Work out the finished part from the listing and answer in its coordinate system (mm). Coordinates: 2 decimals unless noted, no trailing zeros. Write each loop counter-clockwise with the first axis right and the second up, starting at its lowest first coordinate (ties: lowest second). Pieces come first, ordered by that corner, then holes. Notation, with made-up numbers: (-27, 17.25) - (4, 17.25) arc R5 cw to (4, 26.25) - close; hole circle Ø9 at (50.5, 54.25). An arc over 180 degrees is marked (long way). Use a Markdown table: item, result. Add a question column.
(1) The part is cut by section A-A, the plane z = 38.1. Give the vertices of the cut face in (x, y) (3 decimals).
(2) For a pull along X with two mould halves and no side action, classify faces 1 (the face through (-15.075, -0.044, -1.252)), 2 (the face through (-19, 0, -57.15)), 3 (the face through (38.1, 0, 38)), 4 (the face through (-19.592, -0.044, -42.232)) as released by +X, released by -X, zero draft, split by the parting line, or undercut.
(3) The part is cut by section C-C, the plane y = 0. Give the vertices of the cut face in (x, z).
(4) Find the intervals of material crossed by line 1 (Z direction, x = -19.05, y = 1); line 2 (X direction, y = -0.5, z = 38.1); line 3 (Z direction, x = -21, y = -1.5), in increasing order. Write a range as from..to.
(5) The part is cut by section B-B, the plane x = -19.05. Give the vertices of the cut face in (y, z) (3 decimals).
(6) The part is cut by section D-D, the plane x = 19.05. Give the vertices of the cut face in (y, z) (3 decimals), then the cut area to 3 significant figures.
(7) Given pin 1 Ø3 at (x, y) = (13.5, -1.5) entering from -Z; pin 2 Ø3 at (y, z) = (0, -25) entering from +X (3 decimals), each flat-ended and moving along its own axis, determine where each tip first touches the part or whether it passes through.
from build123d import *

# Parameters (mm, degrees)
SKETCH1_W           = 76.2
SKETCH1_H           = 6.35
BOSS_EXTRUDE1_DEPTH = 57.15
CUT_EXTRUDE3_DEPTH  = 7.62
LPATTERN1_START     = -3.175
LPATTERN1_OUTLINE_R = 4.167251
LPATTERN1_DEPTH     = 6.35


# Read off the part's stored shape, not the designer's step: LPattern1
with BuildPart() as part:
    # Sketch1 → Boss-Extrude1 (new, symmetric)
    with BuildSketch(Plane.XY):
        Rectangle(SKETCH1_W, SKETCH1_H)
    extrude(amount=BOSS_EXTRUDE1_DEPTH, both=True)

    # Sketch8 → Cut-Extrude3 (cut)
    with BuildSketch(Plane(origin=(0, 3.175, 0), x_dir=(-1, 0, 0), z_dir=(0, 1, 0))):
        Polygon((0, -57.15), (-38.1, 19.05), (-38.1, -57.15), align=None)
    extrude(amount=-CUT_EXTRUDE3_DEPTH, mode=Mode.SUBTRACT)

    # Sketch9 → 21_64 _0.32813_ Diameter Hole1 (revolve, cut)
    with BuildSketch(Plane(origin=(-19.05, 3.175, 38.1), x_dir=(0, 0, 1), z_dir=(1, 0, 0))):
        Polygon((0, 0), (0, 8.853937016), (4.167251, 6.35), (4.167251, 0), align=None)
    revolve(axis=Axis((-19.05, 9.525, 38.1), (0, -1, 0)), mode=Mode.SUBTRACT)

    # LPattern1 outline → LPattern1 (cut)
    with BuildSketch(Plane(origin=(0, 0, 0), x_dir=(1, 0, 0), z_dir=(0, 1, 0)).offset(LPATTERN1_START)):
        with Locations((19.05, -38.1)):
            Circle(LPATTERN1_OUTLINE_R)
        with Locations((-19.05, 0)):
            Circle(LPATTERN1_OUTLINE_R)
        with Locations((-19.05, 38.1)):
            Circle(LPATTERN1_OUTLINE_R)
    extrude(amount=LPATTERN1_DEPTH, mode=Mode.SUBTRACT)


solid = part.part
Model answer:
| question | item | result |
|---|---|---|
| 1 | outline | (-38.1, -3.175) - (-23.217, -3.175) - (-23.217, 3.175) - (-38.1, 3.175) - close; (-14.883, -3.175) - (14.883, -3.175) - (14.883, 3.175) - (-14.883, 3.175) - close; (23.217, -3.175) - (38.1, -3.175) - (38.1, 3.175) - (23.217, 3.175) - close |
| 2 | face 1 | undercut |
| 2 | face 2 | zero draft |
| 2 | face 3 | released by +X |
| 2 | face 4 | undercut |
| 3 | outline | (-38.1, -57.15) - (0, -57.15) - (38.1, 19.05) - (38.1, 57.15) - (-38.1, 57.15) - close; hole circle Ø8.33 at (-19.05, -38.1); hole circle Ø8.33 at (-19.05, 0); hole circle Ø8.33 at (-19.05, 38.1); hole circle Ø8.33 at (19.05, 38.1) |
| 4 | line 1 | -57.15..-42.27, -33.93..-4.17, 4.17..33.93, 42.27..57.15 |
| 4 | line 2 | -38.1..-23.22, -14.88..14.88, 23.22..38.1 |
| 4 | line 3 | -57.15..-41.78, -34.42..-3.68, 3.68..34.42, 41.78..57.15 |
| 5 | outline | (-3.175, -57.15) - (3.175, -57.15) - (3.175, -42.267) - (-3.175, -42.267) - close; (-3.175, -33.933) - (3.175, -33.933) - (3.175, -4.167) - (-3.175, -4.167) - close; (-3.175, 4.167) - (3.175, 4.167) - (3.175, 33.933) - (-3.175, 33.933) - close; (-3.175, 42.267) - (3.175, 42.267) - (3.175, 57.15) - (-3.175, 57.15) - close |
| 6 | outline | (-3.175, -19.05) - (3.175, -19.05) - (3.175, 33.933) - (-3.175, 33.933) - close; (-3.175, 42.267) - (3.175, 42.267) - (3.175, 57.15) - (-3.175, 57.15) - close |
| 6 | area | 431 mm^2 |
| 7 | pin 1 | z = -33.15 |
| 7 | pin 2 | x = 16.825 |
